Check sheet for the drawn part. Datum: minimum x, y, z corner. Units: mm. Round coordinates to 2 decimals unless told otherwise and drop trailing zeros. Order: outer loops, then holes, each group sorted by start corner. A loop starts at its lowest first (then second) coordinate and runs counter-clockwise, first axis right, second up.
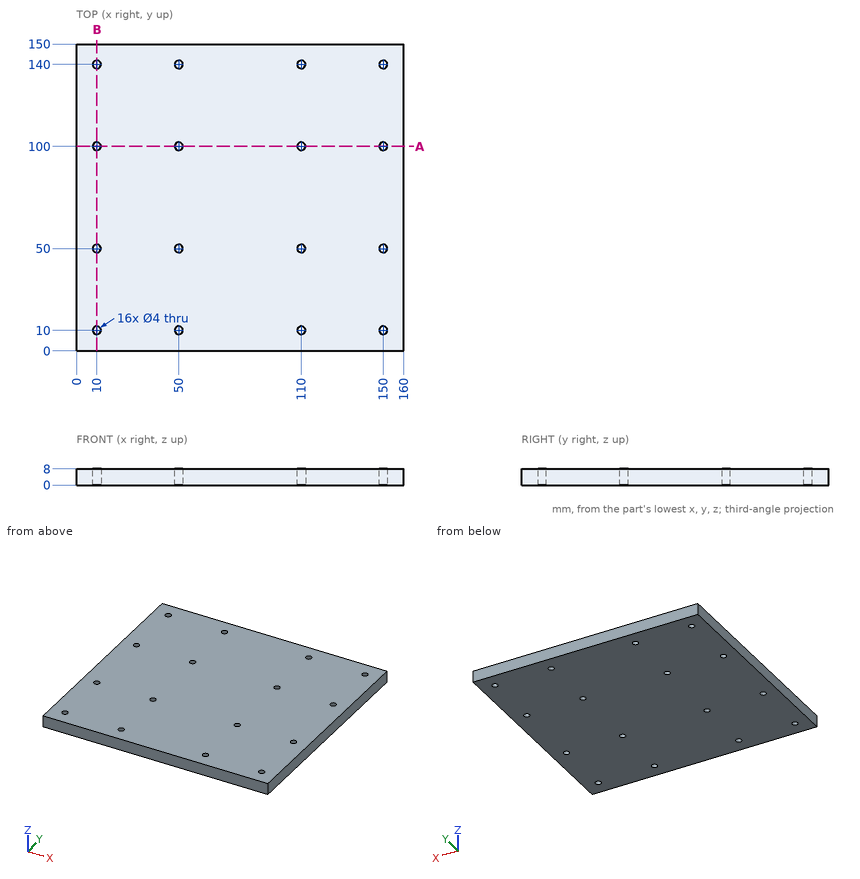
(1) Sectioned sample at B-B, the plane x = 10. Record the cut outline in (y, z).
Returned:
outline: (0, 0) - (8, 0) - (8, 8) - (0, 8) - close; (12, 0) - (48, 0) - (48, 8) - (12, 8) - close; (52, 0) - (98, 0) - (98, 8) - (52, 8) - close; (102, 0) - (138, 0) - (138, 8) - (102, 8) - close; (142, 0) - (150, 0) - (150, 8) - (142, 8) - close
(2) Material ranges on line 1 (Y direction, x = 10, z = 5); line 2 (X direction, y = 100, z = 3); line 3 (Y direction, x = 148.5, z = 4.5), recorded low to high.
Returned:
line 1: y = 0 to 8, 12 to 48, 52 to 98, 102 to 138, 142 to 150
line 2: x = 0 to 8, 12 to 48, 52 to 108, 112 to 148, 152 to 160
line 3: y = 0 to 8.68, 11.32 to 48.68, 51.32 to 98.68, 101.32 to 138.68, 141.32 to 150
(3) Depth check by flat-ended pin: P1, Ø3, axis at x = 50, y = 100, coming from the -Z side. Enter the tip coordinate at first touch or a pass-through.
Returned:
P1: passes through
(4) Sectioned sample at A-A, the plane y = 100. Record the cut outline in (x, z).
Returned:
outline: (0, 0) - (8, 0) - (8, 8) - (0, 8) - close; (12, 0) - (48, 0) - (48, 8) - (12, 8) - close; (52, 0) - (108, 0) - (108, 8) - (52, 8) - close; (112, 0) - (148, 0) - (148, 8) - (112, 8) - close; (152, 0) - (160, 0) - (160, 8) - (152, 8) - close
